Answer from the drawing. Dimensions are ordinates in mm from the lowest x, y and z of the part. Coordinates: 2 decimals unless noted, no trailing zeros. Write each loop counter-clockwise with the first axis right and the second up, starting at its lowest first coordinate (ties: lowest second). Pieces come first, ordered by that corner, then holes. Notation, with made-up numbers: (-38.5, -34) - (-12.5, -34) arc R22 cw to (-12.5, 5) - close; hole circle Ø8 at (85.25, 25). An arc over 180 degrees is marked (long way). Use a Markdown table: item, result.
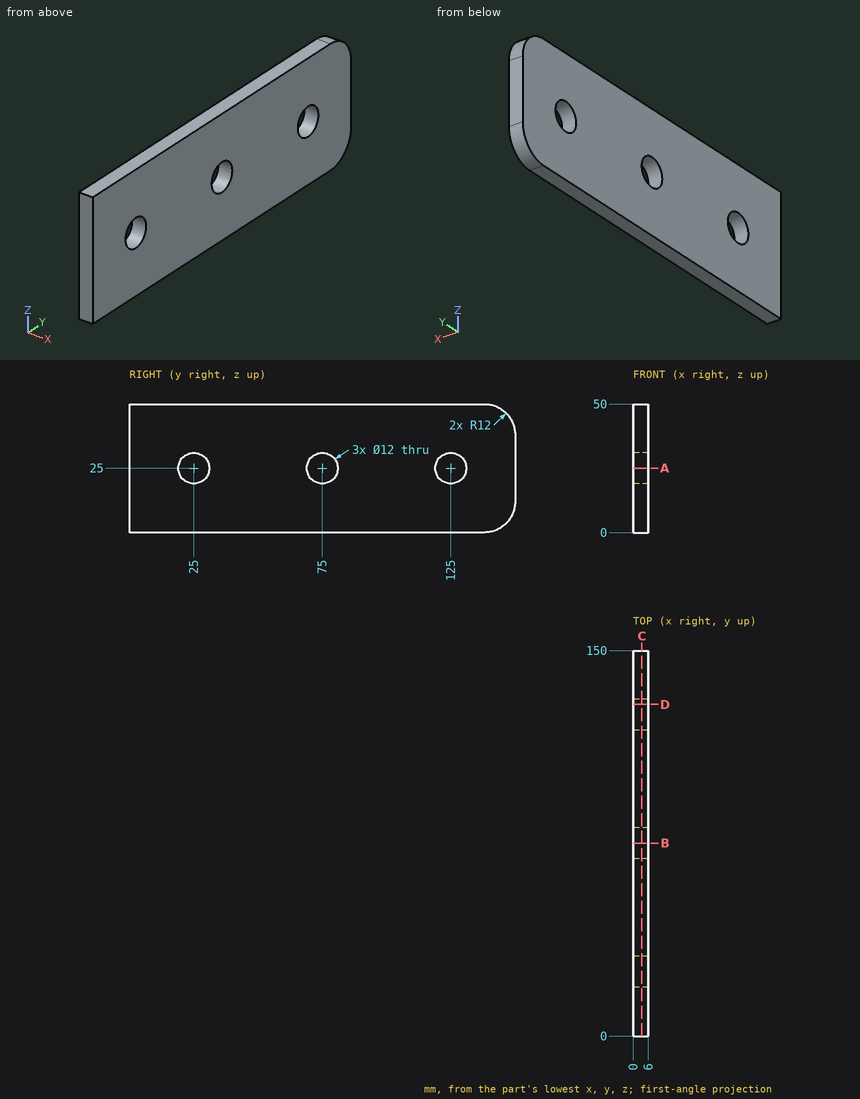
(1) This flat-tipped pin is pushed along its axis until it touches: P1, Ø9.5, axis at y = 75, z = 25, coming from the +X side. Where does it stop, or does it pass through?
Report:
| item | result |
|---|---|
| P1 | passes through |
(2) Straight lines are drawn through the part: L1, parallel to Y at x = 2.6, z = 25; L2, parallel to Z at x = 4.3, y = 125; L3, parallel to Y at x = 5.25, z = 19.5. For each, find the intervals that lie inside material, in ascending order.
Report:
| item | result |
|---|---|
| L1 | y = 0 to 19, 31 to 69, 81 to 119, 131 to 150 |
| L2 | z = 0 to 19, 31 to 50 |
| L3 | y = 0 to 22.6, 27.4 to 72.6, 77.4 to 122.6, 127.4 to 150 |
(3) A cutting plane is placed at D-D, the plane y = 129. Write down the section's boundary in (x, z).
Report:
| item | result |
|---|---|
| outline | (0, 0) - (6, 0) - (6, 20.53) - (0, 20.53) - close; (0, 29.47) - (6, 29.47) - (6, 50) - (0, 50) - close |
(4) A cutting plane is placed at A-A, the plane z = 25. Write down the section's boundary in (x, y).
Report:
| item | result |
|---|---|
| outline | (0, 0) - (6, 0) - (6, 19) - (0, 19) - close; (0, 31) - (6, 31) - (6, 69) - (0, 69) - close; (0, 81) - (6, 81) - (6, 119) - (0, 119) - close; (0, 131) - (6, 131) - (6, 150) - (0, 150) - close |
(5) A cutting plane is placed at B-B, the plane y = 75. Write down the section's boundary in (x, z), and give its area (3 significant figures).
Report:
| item | result |
|---|---|
| outline | (0, 0) - (6, 0) - (6, 19) - (0, 19) - close; (0, 31) - (6, 31) - (6, 50) - (0, 50) - close |
| area | 228 mm² |
(6) A cutting plane is placed at C-C, the plane x = 3.45. Write down the section's boundary in (y, z).
Report:
| item | result |
|---|---|
| outline | (0, 0) - (138, 0) arc R12 ccw to (150, 12) - (150, 38) arc R12 ccw to (138, 50) - (0, 50) - close; hole circle Ø12 at (25, 25); hole circle Ø12 at (75, 25); hole circle Ø12 at (125, 25) |
